Geometry check sheet. Reference: drawing and pictorial views, mm from the part's lowest x, y, z. Round coordinates to 2 decimals unless told otherwise and drop trailing zeros. Loops run counter-clockwise (first coordinate to the right, second up) from the corner with the lowest first, then second, coordinate; pieces in that order, holes last. Notation, with made-up numbers: M 12.25,37 L 40.25,37 A9 cw 40.25,48 Z; hole C 6,52.25 d8. An arc over 180 degrees is marked long. One line per question, with ' | ' between items. Start each with the question number.
(1) Thickness scan on probe 1 along X at (y, z) = (0.6, 40); probe 2 along X at (y, z) = (0.7, 37.5); probe 3 along Z at (x, y) = (40, 0.4). Record the ranges inside material, lowest first. Write a range as [from, to].
(2) Section check B-B (y = 0.45). Record the boundary of the cut face in (x, z).
(3) Section check C-C (z = 40). Record the boundary of the cut face in (x, y).
(4) Section check A-A (x = 40). Record the boundary of the cut face in (y, z), and give its area (3 significant figures).
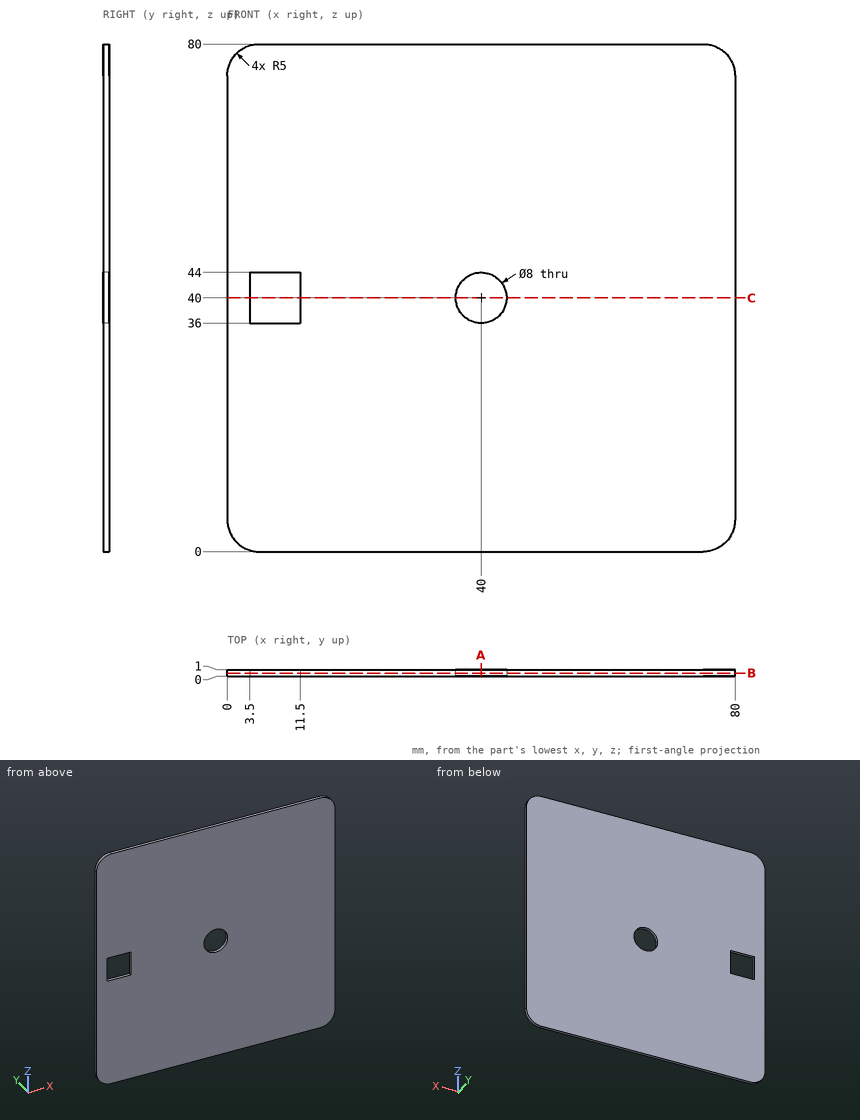
The answers:
1) probe 1: [0, 3.5], [11.5, 36], [44, 80] | probe 2: [0, 3.5], [11.5, 36.88], [43.12, 80] | probe 3: [0, 36], [44, 80]
2) outline: M 0,5 A5 ccw 5,0 L 75,0 A5 ccw 80,5 L 80,75 A5 ccw 75,80 L 5,80 A5 ccw 0,75 Z; hole M 3.5,36 L 11.5,36 L 11.5,44 L 3.5,44 Z; hole C 40,40 d8
3) outline: M 0,0 L 3.5,0 L 3.5,1 L 0,1 Z; M 11.5,0 L 36,0 L 36,1 L 11.5,1 Z; M 44,0 L 80,0 L 80,1 L 44,1 Z
4) outline: M 0,0 L 1,0 L 1,36 L 0,36 Z; M 0,44 L 1,44 L 1,80 L 0,80 Z | area: 72.0 mm²
